For this review, take the finished solid that the model builds, in its own axes (mm). Give positions to 0.01 mm unless a question says otherwise; leave off trailing zeros. Order: outer loops, then holes, each group sorted by start corner. A loop starts at its lowest first (then second) coordinate and runs counter-clockwise, first axis right, second up.
Autodesk Inventor part; units mm, degrees
ref_plane "YZ Plane" through (0, 0, 0) normal (1, 0, 0) x (0, 1, 0)
ref_plane "XZ Plane" through (0, 0, 0) normal (0, 1, 0) x (-1, 0, 0)
ref_plane "XY Plane" through (0, 0, 0) normal (0, 0, 1) x (1, 0, 0)
sketch "スケッチ1" plane through (0, 0, 0) normal (1, 0, 0) x (0, 1, 0)
  line L0 (0, 250) -> (114.6125, -400)
  line L1 (0, 387.8164) -> (0, -558.8236)
  arc A0 (0, 250) -> (21.0831, -240) centre (1567.8058, 72.0039) ccw
  arc A1 (21.0831, -240) -> (114.6125, -400) centre (301.453, -183.444) ccw
  arc A2 (0, 250) -> (-64.6034, 4.1758) centre (731.6003, -73.6681) ccw
  arc A3 (-64.6034, 4.1758) -> (114.6125, -400) centre (382.2372, -39.5113) ccw
  point P0 (0, 0)
  dimension "d0" = 10
  dimension "d1" = 650
  dimension "d4" = 250
  dimension "d10" = 1577.8776
  dimension "d11" = 286.0172
  dimension "d12" = 160
  dimension "d13" = 800
extrude "押し出し2" add sketch "スケッチ1" along normal mid plane 950 contours A0 L1 A3 A2 | A3 L1 A0 A1
fillet "フィレット3" radius 10 1 edges at (0, 0, 250)
fillet "フィレット3" radius 2 1 edges at (0, 114.6125, -400)
properties part number "cover_re" material "ポリスチレン"
1) To check wall thickness, follow line 1 (Z direction, x = -184, y = 66.5); line 2 (Y direction, x = 310, z = -246); line 3 (Y direction, x = 238.5, z = 23.5). State the ranges of each line that lie inside material, in increasing order.
Answer sheet:
line 1: z = -358.71 to -346.55
line 2: y = -16.43 to 22.36
line 3: y = -62.48 to -9.33
2) We need section B-B on y = 44.5. Give the boundary of the cut face in (x, z), then the cut area to 3 significant figures.
Answer sheet:
outline: (-475, -335.33) - (475, -335.33) - (475, -309.07) - (-475, -309.07) - close
area: 25,000 mm2
3) Clearance check with flat-ended pins moving along their axes: pin 1 (12 mm diameter, centred on x = -59, z = 24, fed in from +Y); pin 2 (6 mm diameter, centred on x = -210, y = -1, fed in from -Z). State where each tip first meets the part, or that it passes through.
Answer sheet:
pin 1: stops at y = -9.15
pin 2: stops at z = -278.25
4) We need section A-A on z = 82. Give the boundary of the cut face in (x, y).
Answer sheet:
outline: (-475, -53.11) - (475, -53.11) - (475, -10.04) - (-475, -10.04) - close
